```python
from build123d import *

# Parameters (mm, degrees)
F0_W = 1.27
F0_H = 6.35
F2_R = 0.508
F5_R = 0.254


with BuildPart() as f1:
    # F0 (on Front) → F1 (revolve)
    with BuildSketch(Plane.XZ):
        with Locations((0.635, 3.683)):
            Rectangle(F0_W, F0_H)
    revolve(axis=Axis((0, 0, 3.683), (0, 0, 1)))

    # F2
    f2_edges = [f1.edges().sort_by_distance(p)[0] for p in [
        (-1.27, 0, 6.858),
        (-1.27, 0, 0.508),
    ]]
    fillet(f2_edges, radius=F2_R)

    # F6: sweep along a path in F3
    with BuildLine(Plane.XZ) as f6_path:
        Line((0, -3.81), (0, 7.493))
        ThreePointArc((0, 7.493), (-0.3719743879, 8.3910256121), (-1.27, 8.763))
        Line((-1.27, 8.763), (-3.81, 8.763))
        ThreePointArc((-3.81, 8.763), (-4.7080256121, 8.3910256121), (-5.08, 7.493))
        Line((-5.08, 7.493), (-5.08, -3.81))
    # F5 (on offset) → F6 (sweep)
    with BuildSketch(Plane.XY.offset(-3.81)):
        Circle(F5_R)
    sweep(path=f6_path.line)


solid = f1.part
```
Could you check a few things on this model? Use its own coordinates, in mm. Round coordinates to 2 decimals unless told otherwise and drop trailing zeros. Loops run counter-clockwise (first coordinate to the right, second up) from the corner with the lowest first, then second, coordinate; pieces in that order, holes last. Notation, with made-up numbers: (63.5, -23.75) - (91.5, -23.75) arc R24 ccw to (91.5, -13.75) - close; hole circle Ø8 at (83.25, -16). An arc over 180 degrees is marked (long way). Answer as CSV lines item,"result".
1. I want a section at A-A on z = 2.25. List the corners of the cut face in (x, y) for me, then the cut area to 3 significant figures.
Filled in:
outline,"circle Ø0.51 at (-5.08, 0); circle Ø2.54 at (0, 0)"
area,"5.27 mm^2"
2. I want a section at B-B on y = 0. List the corners of the cut face in (x, z) for me, then the cut area to 3 significant figures.
Filled in:
outline,"(-5.33, -3.81) - (-4.83, -3.81) - (-4.83, 7.49) arc R1.02 cw to (-3.81, 8.51) - (-1.27, 8.51) arc R1.02 cw to (-0.25, 7.49) - (-0.25, 6.86) - (-0.76, 6.86) arc R0.51 ccw to (-1.27, 6.35) - (-1.27, 1.02) arc R0.51 ccw to (-0.76, 0.51) - (-0.25, 0.51) - (-0.25, -3.81) - (0.25, -3.81) - (0.25, 0.51) - (0.76, 0.51) arc R0.51 ccw to (1.27, 1.02) - (1.27, 6.35) arc R0.51 ccw to (0.76, 6.86) - (0.25, 6.86) - (0.25, 7.49) arc R1.52 ccw to (-1.27, 9.02) - (-3.81, 9.02) arc R1.52 ccw to (-5.33, 7.49) - close"
area,"27.5 mm^2"
3. Please list where these lines run through material, in increasing order: line 1 along Z through (x, y) = (0, 0.4); line 2 along X through (y, z) = (-0.1, 0); line 3 along Z through (x, y) = (1, -0.3). Write a range as [from, to].
Filled in:
line 1,"z = [0.51, 6.86]"
line 2,"x = [-5.31, -4.85], [-0.23, 0.23]"
line 3,"z = [0.59, 6.77]"
4. I want a section at C-C on x = -3.5. List the corners of the cut face in (y, z) for me, then the cut area to 3 significant figures.
Filled in:
outline,"circle Ø0.51 at (0, 8.76)"
area,"0.203 mm^2"
5. I want a section at D-D on z = -1.5. List the corners of the cut face in (x, y) for me, then the cut area to 3 significant figures.
Filled in:
outline,"circle Ø0.51 at (-5.08, 0); circle Ø0.51 at (0, 0)"
area,"0.405 mm^2"
